Could you check a few things on this model? Use its own coordinates, in mm. A direction names the side the tool comes from. Give positions to 0.01 mm unless a question says otherwise; leave off trailing zeros. Write each loop counter-clockwise with the first axis right and the second up, starting at its lowest first coordinate (ties: lowest second). Pieces come first, ordered by that corner, then holes. Notation, with made-up numbers: (29, 76) - (86, 76) arc R22 cw to (86, 88) - close; hole circle Ø3 at (23, 87.25). An arc over 180 degrees is marked (long way). Answer in a Markdown table with one row per item.
from build123d import *

# Parameters (mm, degrees)
F0_W      = 13
F0_H      = 13
F1_DEPTH  = 50
F2_W      = 13
F2_H      = 13
F3_DEPTH  = 50
F5_R      = 1.6
F6_DEPTH  = 25
F8_D      = 6
F9_W      = 13
F9_H      = 5
F10_DEPTH = 20
F11_W     = 4
F11_H     = 13
F12_DEPTH = 36.5
F15_D     = 6.7564
F17_DEPTH = 4
F18_W     = 10
F18_H     = 10
F19_DEPTH = 10
F22_R     = 5
F23_D     = 4
F23_DEPTH = 39
F23_TIP   = 1.2017212381
F24_D     = 4.1
F24_DEPTH = 70
F24_TIP   = 1.231764269


with BuildPart() as f1:
    # F0 (on Front) → F1 (new body)
    with BuildSketch(Plane.XZ):
        Rectangle(F0_W, F0_H)
    extrude(amount=F1_DEPTH)

    # F2 (on face) → F3 (join)
    with BuildSketch(Plane.YZ.offset(6.5)):
        with Locations((-43.5, 0)):
            Rectangle(F2_W, F2_H)
    extrude(amount=F3_DEPTH)

    # F5 (on face) → F6 (join)
    with BuildSketch(Plane(origin=(0, 0, 0), x_dir=(-1, 0, 0), z_dir=(0, 1, 0))):
        Circle(F5_R)
    extrude(amount=F6_DEPTH)

    # F8 (through all)
    with Locations(Plane.XY.offset(6.5)):
        with Locations((0, -28.5), (0, -13.5), (0, -43.5), (15, -43.5), (46.5, -43.5)):
            Hole(F8_D / 2)

    # F9 (on face) → F10 (join)
    with BuildSketch(Plane.YZ.offset(56.5)):
        with Locations((-43.5, 4)):
            Rectangle(F9_W, F9_H)
    extrude(amount=F10_DEPTH)

    # F11 (on face) → F12 (join)
    with BuildSketch(Plane(origin=(0, 0, -6.5), x_dir=(1, 0, 0), z_dir=(0, 0, -1))):
        with Locations((54.5, 43.5)):
            Rectangle(F11_W, F11_H)
    extrude(amount=F12_DEPTH)

    # F15 (through all)
    with Locations(Plane.XY.offset(6.5)):
        with Locations((68.5, -43)):
            Hole(F15_D / 2)

    # F16 (on face) → F17 (cut, through all)
    with BuildSketch(Plane.YZ.offset(56.5)):
        with BuildLine():
            Line((-49.35, -39.3), (-49.35, -40.3))
            ThreePointArc((-49.35, -40.3), (-48.25, -41.4), (-47.15, -40.3))
            Line((-47.15, -40.3), (-47.15, -39.3))
            ThreePointArc((-47.15, -39.3), (-48.25, -38.2), (-49.35, -39.3))
        make_face()
        with BuildLine():
            Line((-49.35, -28.3), (-49.35, -29.3))
            ThreePointArc((-49.35, -29.3), (-48.25, -30.4), (-47.15, -29.3))
            Line((-47.15, -29.3), (-47.15, -28.3))
            ThreePointArc((-47.15, -28.3), (-48.25, -27.2), (-49.35, -28.3))
        make_face()
    extrude(amount=-F17_DEPTH, mode=Mode.SUBTRACT)

    # F18 (on face) → F19 (cut)
    with BuildSketch(Plane.XY.offset(6.5)):
        with Locations((57.5, -43.5)):
            Rectangle(F18_W, F18_H)
    extrude(amount=-F19_DEPTH, mode=Mode.SUBTRACT)

    # F22
    f22_edges = [f1.edges().sort_by_distance(p)[0] for p in [
        (-6.5, -50, 0),
    ]]
    fillet(f22_edges, radius=F22_R)

    # F23
    with Locations(Plane(origin=(0, 0, 0), x_dir=(-1, 0, 0), z_dir=(0, 1, 0))):
        with Locations((-6.5, 0)):
            Hole(F23_D / 2, depth=F23_DEPTH)
            with Locations((0, 0, -(F23_DEPTH + F23_TIP / 2))):  # 118° drill point
                Cone(0, F23_D / 2, F23_TIP, mode=Mode.SUBTRACT)

    # F24
    with Locations(Plane.YZ.offset(76.5)):
        with Locations((-37, 0)):
            Hole(F24_D / 2, depth=F24_DEPTH)
            with Locations((0, 0, -(F24_DEPTH + F24_TIP / 2))):  # 118° drill point
                Cone(0, F24_D / 2, F24_TIP, mode=Mode.SUBTRACT)


solid = f1.part
1) We'd pull the mould along X, two halves only. Please class faces 1 (the face through (6.5, -18, 4)), 2 (the face through (65.379, -44.294, 3.965)), 3 (the face through (54, -43, -3.5)): +X half, -X half, draft (parallel to the pull), parting line (faces both ways), or undercut.
Check values:
| item | result |
|---|---|
| face 1 | +X half |
| face 2 | undercut |
| face 3 | draft |
2) Will these pins go through, and if not, where does the flat tip stop? P1, Ø8, axis at x = 0, y = -13.5, coming from the -Z side; P2, Ø10, axis at x = 44, z = -24.5, coming from the +Y side; P3, Ø1.3, axis at y = -25, z = -5, coming from the +X side; P4, Ø4, axis at y = -37, z = -36.5, coming from the +X side.
Check values:
| item | result |
|---|---|
| P1 | stops at z = -6.5 |
| P2 | passes through |
| P3 | stops at x = 6.5 |
| P4 | stops at x = 56.5 |
3) Imagine slicing it at D-D (z = -36.5). List the corners of the cut face in (x, y) for me.
Check values:
| item | result |
|---|---|
| outline | (52.5, -50) - (56.5, -50) - (56.5, -37) - (52.5, -37) - close |
4) Imagine slicing it at A-A (x = 68.5). List the corners of the cut face in (y, z) for me, then the cut area to 3 significant figures.
Check values:
| item | result |
|---|---|
| outline | (-50, 1.5) - (-46.38, 1.5) - (-46.38, 6.5) - (-50, 6.5) - close; (-39.62, 1.5) - (-38.4, 1.5) arc R2.05 cw to (-37, 2.05) - (-37, 6.5) - (-39.62, 6.5) - close |
| area | 30.7 mm2 |
5) If I drill on line 1 (Y direction, x = 0, z = 2); line 2 (Y direction, x = 68.5, z = 4.4); line 3 (Y direction, x = 15, z = 0), over which ranges is the centre line in solid material (lowest first)?
Check values:
| item | result |
|---|---|
| line 1 | y = -50 to -46.5, -40.5 to -31.5, -25.5 to -16.5, -10.5 to 0 |
| line 2 | y = -50 to -46.38, -39.62 to -37 |
| line 3 | y = -50 to -46.5, -40.5 to -39.05 |
6) Imagine slicing it at C-C (x = 0). List the corners of the cut face in (y, z) for me.
Check values:
| item | result |
|---|---|
| outline | (-50, -6.5) - (-46.5, -6.5) - (-46.5, 6.5) - (-50, 6.5) - close; (-40.5, -6.5) - (-31.5, -6.5) - (-31.5, 6.5) - (-40.5, 6.5) - close; (-25.5, -6.5) - (-16.5, -6.5) - (-16.5, 6.5) - (-25.5, 6.5) - close; (-10.5, -6.5) - (0, -6.5) - (0, -1.6) - (25, -1.6) - (25, 1.6) - (0, 1.6) - (0, 6.5) - (-10.5, 6.5) - close |
7) Imagine slicing it at B-B (y = -28.5). List the corners of the cut face in (x, z) for me.
Check values:
| item | result |
|---|---|
| outline | (-6.5, -6.5) - (-3, -6.5) - (-3, 6.5) - (-6.5, 6.5) - close; (3, -6.5) - (6.5, -6.5) - (6.5, -2) arc R2 cw to (6.5, 2) - (6.5, 6.5) - (3, 6.5) - close |
8) On a 3-axis mill with a long thin cutter (end or side, diameter ignored), from which of +Z, -Z, +X, -X, +Y, -Y can I reach the whole of each face in a straight line? I mean faces 4 (the face through (54.5, -48.2, -27.2)), 5 (the face through (57, -38.5, 4)), 6 (the face through (3, -31, -6.5)), 7 (the face through (6.5, -18, -4)), 8 (the face through (33.23, -39.05, -0.05)). Say none if no direction works.
Check values:
| item | result |
|---|---|
| face 4 | +X, -X |
| face 5 | +Z |
| face 6 | -Z, -X, +Y, -Y |
| face 7 | +Z, -Z, +X, +Y |
| face 8 | +X, +Y |
